Work out the finished part from the listing and answer in its coordinate system (mm). A direction names the side the tool comes from. Give positions to 0.01 mm unless a question says otherwise; leave off trailing zeros. Loops run counter-clockwise (first coordinate to the right, second up) from the corner with the lowest first, then second, coordinate; pieces in that order, holes last. Notation, with made-up numbers: (58, 87) - (115, 87) arc R28 cw to (115, 114) - close; hole circle Ø10 at (72, -6). An arc over 180 degrees is marked (long way). One line per item, written item: value.
from build123d import *

# Parameters (mm, degrees)
SKETCH1_R           = 1.5
SKETCH1_W           = 125
SKETCH1_H           = 124.954514062
SKETCH1_W_2         = 5
SKETCH1_H_2         = 5
BOSS_EXTRUDE1_DEPTH = 5
FILLET1_R           = 10


with BuildPart() as part:
    # Sketch1 → Boss-Extrude1 (new body)
    with BuildSketch(Plane.XY):
        Polygon((92.5, 62.5), (92.5, -62.5), (92.5, -65), (97.5, -65), (97.5, -70), (92.5, -70), (92.5, -73.5), (89.5, -73.5), (89.5, -72.4), (87.2, -72.4), (87.2, -73.5), (82.5, -73.5), (82.5, -76.5), (87.2, -76.5), (87.2, -77.6), (89.5, -77.6), (89.5, -76.5), (92.5, -76.5), (92.5, -80), (97.5, -80), (97.5, -85), (92.5, -85), (92.5, -90), (-92.5, -90), (-92.5, -85), (-97.5, -85), (-97.5, -80), (-92.5, -80), (-92.5, -76.5), (-89.5, -76.5), (-89.5, -77.6), (-87.2, -77.6), (-87.2, -76.5), (-82.5, -76.5), (-82.5, -73.5), (-87.2, -73.5), (-87.2, -72.4), (-89.5, -72.4), (-89.5, -73.5), (-92.5, -73.5), (-92.5, -70), (-97.5, -70), (-97.5, -65), (-92.5, -65), (-92.5, 65), (-97.5, 65), (-97.5, 70), (-92.5, 70), (-92.5, 73.5), (-89.5, 73.5), (-89.5, 72.4), (-87.2, 72.4), (-87.2, 73.5), (-82.5, 73.5), (-82.5, 76.5), (-87.2, 76.5), (-87.2, 77.6), (-89.5, 77.6), (-89.5, 76.5), (-92.5, 76.5), (-92.5, 80), (-97.5, 80), (-97.5, 85), (-92.5, 85), (-92.5, 90), (92.5, 90), (92.5, 85), (97.5, 85), (97.5, 80), (92.5, 80), (92.5, 76.5), (89.5, 76.5), (89.5, 77.6), (87.2, 77.6), (87.2, 76.5), (82.5, 76.5), (82.5, 73.5), (87.2, 73.5), (87.2, 72.4), (89.5, 72.4), (89.5, 73.5), (92.5, 73.5), (92.5, 70), (97.5, 70), (97.5, 65), (92.5, 65), align=None)
        with Locations((60, 82.5)):
            Circle(SKETCH1_R, mode=Mode.SUBTRACT)
        with Locations((-60, -82.5)):
            Circle(SKETCH1_R, mode=Mode.SUBTRACT)
        with Locations(Location((-60, 82.5, 0), (0, 0, 180))):
            Circle(SKETCH1_R, mode=Mode.SUBTRACT)
        with Locations(Location((30.537723616, -82.5, 0), (0, 0, 90))):
            Circle(SKETCH1_R, mode=Mode.SUBTRACT)
        Rectangle(SKETCH1_W, SKETCH1_H, mode=Mode.SUBTRACT)
        with Locations((52.5, 82.5)):
            Rectangle(SKETCH1_W_2, SKETCH1_H_2, mode=Mode.SUBTRACT)
        with Locations((67.5, 82.5)):
            Rectangle(SKETCH1_W_2, SKETCH1_H_2, mode=Mode.SUBTRACT)
        with Locations((-52.5, -82.5)):
            Rectangle(SKETCH1_W_2, SKETCH1_H_2, mode=Mode.SUBTRACT)
        with Locations((-67.5, -82.5)):
            Rectangle(SKETCH1_W_2, SKETCH1_H_2, mode=Mode.SUBTRACT)
        with Locations((-52.5, 82.5)):
            Rectangle(SKETCH1_W_2, SKETCH1_H_2, mode=Mode.SUBTRACT)
        with Locations((-67.5, 82.5)):
            Rectangle(SKETCH1_W_2, SKETCH1_H_2, mode=Mode.SUBTRACT)
        with Locations((23.037723616, -82.5)):
            Rectangle(SKETCH1_W_2, SKETCH1_H_2, mode=Mode.SUBTRACT)
        with Locations((38.037723616, -82.5)):
            Rectangle(SKETCH1_W_2, SKETCH1_H_2, mode=Mode.SUBTRACT)
    extrude(amount=BOSS_EXTRUDE1_DEPTH)

    # Fillet1
    fillet1_edges = [part.edges().sort_by_distance(p)[0] for p in [
        (62.5, -62.477257031, 2.5),
        (62.5, 62.477257031, 2.5),
        (-62.5, 62.477257031, 2.5),
        (-62.5, -62.477257031, 2.5),
    ]]
    fillet(fillet1_edges, radius=FILLET1_R)


solid = part.part
1. Section C-C (z = 3.95) is taken. Count the separate pieces of the cut face and the enclosed holes in it, and give its area (3 significant figures).
Output:
separate pieces: 1
enclosed holes: 13
area: 17,600 mm²
2. The mould has two halves that part along Y. Classify faces 1 (the flat face through (1, -90, 2)), 2 (the flat face through (20.538, -83, 2)), 3 (the flat face through (-53, 80, 2)), 4 (the flat face through (97.5, -82, 2)): released by +Y, released by -Y, zero draft, split by the parting line, or undercut.
Output:
face 1: released by -Y
face 2: undercut
face 3: undercut
face 4: zero draft
3. Find the intervals of material crossed by line 1 along Y through (x, z) = (53.5, 3.85); line 2 along X through (y, z) = (40.5, 1); line 3 along Y through (x, z) = (47.5, 1), in increasing order.
Output:
line 1: y = -90 to -62.43, 62.43 to 80, 85 to 90
line 2: x = -92.5 to -62.5, 62.5 to 92.5
line 3: y = -90 to -62.48, 62.48 to 90
4. Flat-ended cylindrical pins translate along their axes: pin 1 Ø2 at (y, z) = (26.5, 3.5) entering from +X; pin 2 Ø0.9 at (y, z) = (-77, 3) entering from -X; pin 3 Ø1.5 at (y, z) = (75, 3.5) entering from +X. Find the tip coordinate at first contact, or state that the pin passes through.
Output:
pin 1: stops at x = 92.5
pin 2: stops at x = -92.5
pin 3: stops at x = 82.5
5. For faces 5 (the flat face through (-85, 76.5, 2)), 6 (the flat face through (-92.5, -88, 2)), 7 (the flat face through (-68, -80, 2)), determine the directions among +Z, -Z, +X, -X, +Y, -Y from which every point of the face is accessible in a straight line to the end or side of a thin tool.
Output:
face 5: +Z, -Z, -X
face 6: +Z, -Z, -X, -Y
face 7: +Z, -Z
6. Section A-A (x = -10) is taken. Write down the section's boundary in (y, z), and give its area (3 significant figures).
Output:
outline: (-90, 0) - (-62.48, 0) - (-62.48, 5) - (-90, 5) - close; (62.48, 0) - (90, 0) - (90, 5) - (62.48, 5) - close
area: 275 mm²
7. Section B-B (y = 22.5) is taken. Write down the section's boundary in (x, z).
Output:
outline: (-92.5, 0) - (-62.5, 0) - (-62.5, 5) - (-92.5, 5) - close; (62.5, 0) - (92.5, 0) - (92.5, 5) - (62.5, 5) - close
